Verification items for the finished model (mm, model axes). A direction names the side the tool comes from. Round coordinates to 2 decimals unless told otherwise and drop trailing zeros. Order: outer loops, then holes, each group sorted by start corner. A loop starts at its lowest first (then second) coordinate and runs counter-clockwise, first axis right, second up. Notation, with made-up numbers: (69, 76.25) -> (116, 76.25) arc R28 ccw to (116, 115.25) -> close; hole circle Ø7 at (39.25, -40). An arc over 180 degrees is marked (long way). Return JSON: item names as keys, results as strings. Group by question number.
Item 1: Sectioned sample at B-B on z = 18.5. Record the cut outline in (x, y), plus the area to 3 significant figures.
Item 2: Access from +Z, -Z, +X, -X, +Y, -Y to the whole of each face (thin tool, end or side, straight path). Record for faces 1 (the flat face through (100, 65, 60)), 2 (the flat face through (20, 5, 80)), 3 (the flat face through (105, 70, 70)), 4 (the flat face through (20, 50, 15)), 5 (the flat face through (60, 75, 10)).
Item 3: Sectioned sample at A-A on y = 68. Record the cut outline in (x, z).
Item 4: Sectioned sample at C-C on x = 56. Record the cut outline in (y, z), plus the area to 3 significant figures.
Item 5: Draft check along Z on faces 6 (the flat face through (69, 64, 20)), 7 (the flat face through (89, 60, 40)), 8 (the flat face through (120, 31, 38)), 9 (the flat face through (70, 51, 50)). Enter one of: pulls with the +Z half, pulls with the -Z half, needs draft (parallel to the pull), parting line crosses it, or undercut.
Item 6: Sectioned sample at D-D on y = 47. Record the cut outline in (x, z).
Item 7: Scan lines: probe 1 along Y at (x, z) = (32, 57); probe 2 along Z at (x, y) = (88.5, 75.5); probe 3 along Y at (x, z) = (105.5, 47). Record each from-to range of solid material in increasing order. Write a range as from..to.
Item 8: Depth check by flat-ended pin: pin 1 Ø10 at (x, y) = (11.5, 47.5) entering from +Z; pin 2 Ø10 at (x, z) = (25, 30.5) entering from +Y; pin 3 Ø2 at (y, z) = (35, 76.5) entering from -X; pin 4 Ø8 at (x, y) = (98.5, 66.5) entering from -Z. Enter the tip coordinate at first touch or a pass-through.
```python
from build123d import *

# Parameters (mm, degrees)
SKETCH1_W           = 120
SKETCH1_H           = 80
BOSS_EXTRUDE1_DEPTH = 100
CUT_EXTRUDE1_DEPTH  = 100
CUT_EXTRUDE2_DEPTH  = 100
SKETCH4_W           = 120
SKETCH4_H           = 80
CUT_EXTRUDE3_DEPTH  = 100
CUT_EXTRUDE4_DEPTH  = 10
BOSS_EXTRUDE4_DEPTH = 20
BOSS_EXTRUDE5_DEPTH = 10
CUT_EXTRUDE8_DEPTH  = 156
CUT_EXTRUDE10_DEPTH = 156
CUT_EXTRUDE11_DEPTH = 156
CUT_EXTRUDE12_DEPTH = 156


with BuildPart() as part:
    # Sketch1 → Boss-Extrude1 (new body)
    with BuildSketch(Plane.XY):
        with Locations((60, 40)):
            Rectangle(SKETCH1_W, SKETCH1_H)
    extrude(amount=BOSS_EXTRUDE1_DEPTH)

    # Sketch2 → Cut-Extrude1 (cut)
    with BuildSketch(Plane(origin=(0, 80, 0), x_dir=(1, 0, 0), z_dir=(0, 1, 0))):
        Polygon((0, -60), (40, -100), (0, -100), align=None)
    extrude(amount=-CUT_EXTRUDE1_DEPTH, mode=Mode.SUBTRACT)

    # Sketch3 → Cut-Extrude2 (cut)
    with BuildSketch(Plane(origin=(0, 0, 0), x_dir=(-1, 0, 0), z_dir=(0, 0, -1))):
        Polygon((0, 40), (-30, 70), (-60, 70), (-60, 80), (0, 80), align=None)
    extrude(amount=-CUT_EXTRUDE2_DEPTH, mode=Mode.SUBTRACT)

    # Sketch4 → Cut-Extrude3 (cut)
    with BuildSketch(Plane(origin=(0, 40, 0), x_dir=(1, 0, 0), z_dir=(0, 1, 0))):
        with Locations((60, -60)):
            Rectangle(SKETCH4_W, SKETCH4_H)
    extrude(amount=CUT_EXTRUDE3_DEPTH, mode=Mode.SUBTRACT)

    # Sketch5 → Cut-Extrude4 (cut)
    with BuildSketch(Plane.XY.offset(20)):
        Polygon((20, 40), (20, 60), (0, 40), align=None)
    extrude(amount=-CUT_EXTRUDE4_DEPTH, mode=Mode.SUBTRACT)

    # Sketch6 → Boss-Extrude4 (add)
    with BuildSketch(Plane(origin=(0, 40, 0), x_dir=(1, 0, 0), z_dir=(0, 1, 0))):
        Polygon((40, -20), (120, -20), (120, -80), (100, -80), align=None)
    extrude(amount=BOSS_EXTRUDE4_DEPTH)

    # Sketch8 → Boss-Extrude5 (add)
    with BuildSketch(Plane(origin=(0, 60, 0), x_dir=(1, 0, 0), z_dir=(0, 1, 0))):
        Polygon((80, -60), (120, -60), (120, -80), (100, -80), align=None)
    extrude(amount=BOSS_EXTRUDE5_DEPTH)

    # Sketch9 → Cut-Extrude8 (cut)
    with BuildSketch(Plane(origin=(120, 0, 0), x_dir=(0, 0, -1), z_dir=(1, 0, 0))):
        Polygon((-100, 40), (-80, 40), (-100, 20), align=None)
    extrude(amount=-CUT_EXTRUDE8_DEPTH, mode=Mode.SUBTRACT)

    # Sketch13 → Cut-Extrude10 (cut)
    with BuildSketch(Plane(origin=(-23.333333333, 23.333333333, 23.333333333), x_dir=(0.816496581, 0.40824829, 0.40824829), z_dir=(-0.577350269, 0.577350269, 0.577350269))):
        Polygon((28.577380332, 7.071067812), (28.577380332, -35.355339059), (77.567175188, -63.639610307), (89.814623902, -28.284271247), align=None)
    extrude(amount=CUT_EXTRUDE10_DEPTH, mode=Mode.SUBTRACT)

    # Sketch14 → Cut-Extrude11 (cut)
    with BuildSketch(Plane(origin=(72.619047619, 14.523809524, 58.095238095), x_dir=(-0.605227533, -0.121045507, 0.786795792), z_dir=(-0.77151675, -0.15430335, -0.6172134))):
        Polygon((53.260022875, 1.961161351), (27.840466503, 29.417420271), (51.671300602, 13.237839122), align=None)
    extrude(amount=-CUT_EXTRUDE11_DEPTH, mode=Mode.SUBTRACT)

    # Sketch15 → Cut-Extrude12 (cut)
    with BuildSketch(Plane(origin=(-33.221457258, 0.897877223, 41.302352266), x_dir=(-0.779285755, -0.013620016, -0.626520716), z_dir=(0.626668742, -0.016936993, -0.779101679))):
        Polygon((-94.306519852, 17.821876236), (-92.355669011, 19.098748466), (-93.959701924, 7.824238347), align=None)
    extrude(amount=-CUT_EXTRUDE12_DEPTH, mode=Mode.SUBTRACT)


solid = part.part
```
Recorded:
{
 "1": {"outline": "(0, 0) -> (120, 0) -> (120, 80) -> (60, 80) -> (60, 70) -> (30, 70) -> (20, 60) -> (20, 40) -> (0, 40) -> close", "area": "8,350 mm²"},
 "2": {"face 1": "+X, -X, +Y", "face 2": "+Z, -X, +Y, -Y", "face 3": "+Z, +X, -X, +Y", "face 4": "+Z, -X, +Y", "face 5": "+Z, -Z, -X, +Y"},
 "3": {"outline": "(28, 0) -> (120, 0) -> (120, 20) -> (28, 20) -> close; (80, 60) -> (120, 60) -> (120, 80) -> (100, 80) -> close"},
 "4": {"outline": "(0, 0) -> (70, 0) -> (70, 20) -> (60, 20) -> (60, 36) -> (40, 36) -> (40, 80) -> (20, 100) -> (0, 100) -> close", "area": "4,720 mm²"},
 "5": {"face 6": "undercut", "face 7": "undercut", "face 8": "needs draft", "face 9": "pulls with the +Z half"},
 "6": {"outline": "(7, 0) -> (120, 0) -> (120, 80) -> (100, 80) -> (40, 20) -> (20, 20) -> (20, 10) -> (7, 10) -> close"},
 "7": {"probe 1": "0..40", "probe 2": "0..20", "probe 3": "0..60"},
 "8": {"pin 1": "z = 10", "pin 2": "y = 40", "pin 3": "x = 40.09", "pin 4": "z = 0"}
}
